```python
from build123d import *

# Parameters (mm, degrees)
SZKIC1_W                    = 104
SZKIC1_H                    = 118.94
DODANIE_WYCI_GNI_CIE1_DEPTH = 2
SZKIC2_W                    = 2
SZKIC2_H                    = 118.94
DODANIE_WYCI_GNI_CIE2_DEPTH = 2
SZKIC3_R                    = 1.6
WYTNIJ_WYCI_GNI_CIE1_DEPTH  = 2
ZAOKR_GLENIE1_R             = 2


with BuildPart() as part:
    # Szkic1 → Dodanie-wyciągnięcie1 (new body)
    with BuildSketch(Plane.XY):
        with Locations((-56, 59.47)):
            Rectangle(SZKIC1_W, SZKIC1_H)
    extrude(amount=DODANIE_WYCI_GNI_CIE1_DEPTH)

    # Szkic2 → Dodanie-wyciągnięcie2 (add)
    with BuildSketch(Plane(origin=(0, 0, 0), x_dir=(-1, 0, 0), z_dir=(0, 0, -1))):
        with Locations((109, 59.47)):
            Rectangle(SZKIC2_W, SZKIC2_H)
        with Locations((3, 59.47)):
            Rectangle(SZKIC2_W, SZKIC2_H)
    extrude(amount=-DODANIE_WYCI_GNI_CIE2_DEPTH)

    # Szkic3 → Wytnij-wyciągnięcie1 (cut)
    with BuildSketch(Plane.XY.offset(2)):
        with Locations((-104, 12)):
            Circle(SZKIC3_R)
        with Locations((-8, 12)):
            Circle(SZKIC3_R)
        with Locations((-8, 106.94)):
            Circle(SZKIC3_R)
        with Locations((-104, 106.94)):
            Circle(SZKIC3_R)
    extrude(amount=-WYTNIJ_WYCI_GNI_CIE1_DEPTH, mode=Mode.SUBTRACT)

    # Zaokrąglenie1
    zaokr_glenie1_edges = [part.edges().sort_by_distance(p)[0] for p in [
        (-2, 59.47, 2),
        (-110, 59.47, 2),
    ]]
    fillet(zaokr_glenie1_edges, radius=ZAOKR_GLENIE1_R - 0.0001)  # a hair under: the kernel refuses the full size


solid = part.part
```
Can you work these out from the model? Positions are in its coordinate system, mm. Give positions to 0.01 mm unless a question says otherwise; leave off trailing zeros. Loops run counter-clockwise (first coordinate to the right, second up) from the corner with the lowest first, then second, coordinate; pieces in that order, holes last. Notation, with made-up numbers: M 11.25,5.5 L 46.25,5.5 A16 cw 46.25,28.5 Z; hole C 21,81 d7. An arc over 180 degrees is marked long. Answer in a Markdown table with one row per item.
1. Suppose I cut it at B-B on y = 106.94. Count the separate pieces of the cut face and the enclosed holes in it, plus the area to 3 significant figures.
Taken from the geometry:
| item | result |
|---|---|
| separate pieces | 3 |
| enclosed holes | 0 |
| area | 201 mm² |
2. For pin 1 Ø3 at (x, y) = (-104, 12) entering from +Z, with a flat end and sliding along its axis, tell me the tip position at first contact or that it passes through.
Taken from the geometry:
| item | result |
|---|---|
| pin 1 | passes through |
3. Suppose I cut it at C-C on z = 1.7. Write out the boundary of the cut face in (x, y), plus the area to 3 significant figures.
Taken from the geometry:
| item | result |
|---|---|
| outline | M -109.05,0 L -2.95,0 L -2.95,118.94 L -109.05,118.94 Z; hole C -104,12 d3.2; hole C -104,106.94 d3.2; hole C -8,12 d3.2; hole C -8,106.94 d3.2 |
| area | 12,600 mm² |
4. Thinking about a two-plate mould opening in X: for faces 1 (the cylindrical face through (-105.6, 12.07, 1.01)), 2 (the cylindrical face through (-104.208, 108.526, 1.014)), 3 (the flat face through (-55, 60, 0)), which applies, released by +X, released by -X, zero draft, split by the parting line, or undercut?
Taken from the geometry:
| item | result |
|---|---|
| face 1 | undercut |
| face 2 | undercut |
| face 3 | zero draft |
5. Suppose I cut it at A-A on x = -8. Write out the boundary of the cut face in (y, z), plus the area to 3 significant figures.
Taken from the geometry:
| item | result |
|---|---|
| outline | M 0,0 L 10.4,0 L 10.4,2 L 0,2 Z; M 13.6,0 L 105.34,0 L 105.34,2 L 13.6,2 Z; M 108.54,0 L 118.94,0 L 118.94,2 L 108.54,2 Z |
| area | 225 mm² |
6. If I drill on line 1 along Y through (x, z) = (-8, 0.75); line 2 along X through (y, z) = (107, 1.25); line 3 along X through (y, z) = (106.94, 1.45), over which ranges is the centre line in solid material (lowest first)?
Taken from the geometry:
| item | result |
|---|---|
| line 1 | y = 0 to 10.4, 13.6 to 105.34, 108.54 to 118.94 |
| line 2 | x = -109.56 to -105.6, -102.4 to -9.6, -6.4 to -2.44 |
| line 3 | x = -109.38 to -105.6, -102.4 to -9.6, -6.4 to -2.62 |
